The drawing under review shows one solid part. Ordinate dimensions are in mm from its lowest x, y, z. A direction names the side the tool comes from. Coordinates: 2 decimals unless noted, no trailing zeros. Write each loop counter-clockwise with the first axis right and the second up, starting at its lowest first coordinate (ties: lowest second). Pieces come first, ordered by that corner, then holes.
Q1. To check wall thickness, follow probe 1 along Y at (x, z) = (17.5, 8.5); probe 2 along Z at (x, y) = (12.7, 10.7); probe 3 along Y at (x, z) = (12.7, 2.3). State the ranges of each line that lie inside material, in increasing order.
Q2. Add section B-B, the plane x = 15. Give the boundary of the cut face in (y, z) (3 decimals).
Q3. Add section A-A, the plane z = 6.75. Give the boundary of the cut face in (x, y), plus the area to 3 significant figures.
Q4. Clearance check with flat-ended pins moving along their axes: pin 1 Ø4 at (y, z) = (19.5, 3.5) entering from -X; pin 2 Ø8 at (x, z) = (18.5, 11) entering from +Y; pin 3 Ø3 at (y, z) = (18, 6) entering from +X; pin 4 Ø15 at (x, y) = (18, 22) entering from +Z (3 decimals). State where each tip first meets the part, or that it passes through.
Q5. Machinability: for the marked faces 1, 2 and 3, which of the approach directions +Z, -Z, +X, -X, +Y, -Y give a long, thin tool a straight path to every point of the face, cutting with its end or side? Answer none if there is none.
Q6. Add section D-D, the plane z = 14.25. Give the boundary of the cut face in (x, y).
Q7. The part is to be moulded in two halves that separate along X. For the marked faces 4, 5, 6 and 7, say which applies: +X half, -X half, draft (parallel to the pull), parting line (faces both ways), or undercut.
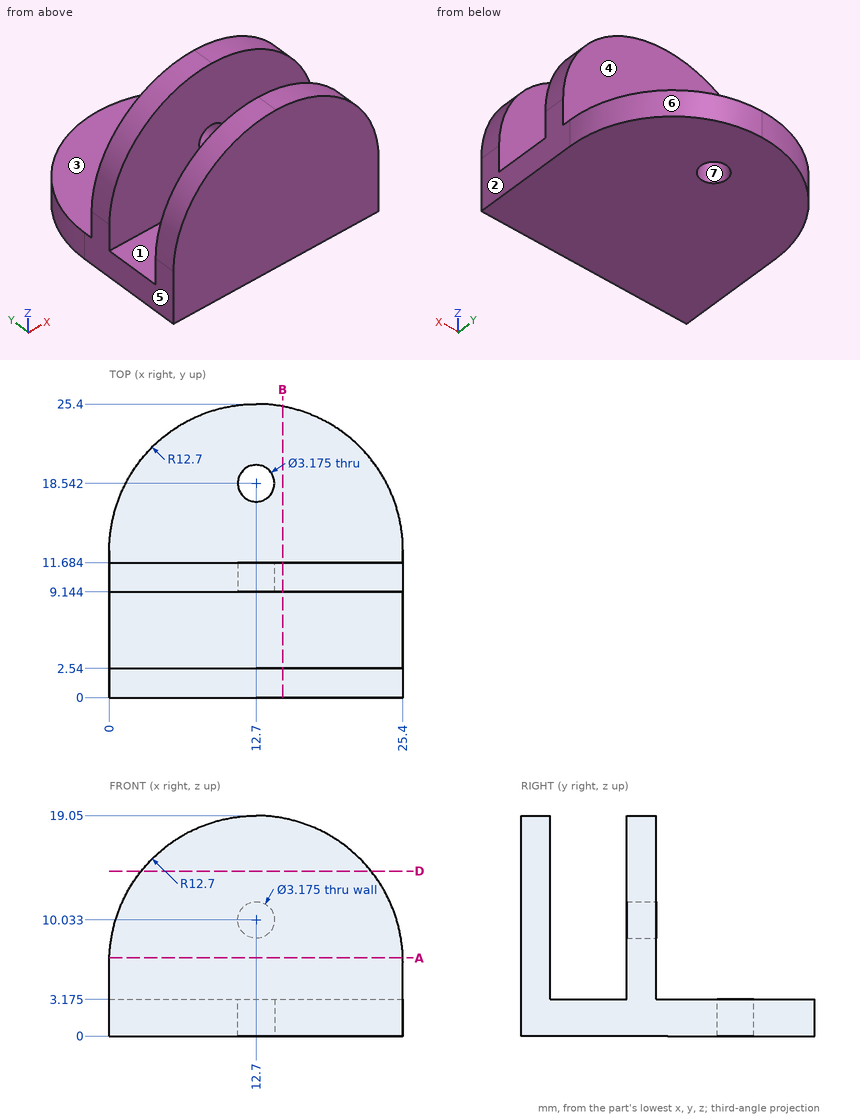
Here are the results:
1. probe 1: y = 0 to 2.54, 9.14 to 11.68
1. probe 2: z = 0 to 8.45, 11.62 to 19.05
1. probe 3: y = 0 to 16.95, 20.13 to 25.4
2. outline: (0, 0) - (25.19, 0) - (25.19, 3.175) - (11.684, 3.175) - (11.684, 18.84) - (9.144, 18.84) - (9.144, 3.175) - (2.54, 3.175) - (2.54, 18.84) - (0, 18.84) - close
3. outline: (0.01, 0) - (25.39, 0) - (25.39, 2.54) - (0.01, 2.54) - close; (0.01, 9.14) - (25.39, 9.14) - (25.39, 11.68) - (0.01, 11.68) - close
3. area: 129 mm2
4. pin 1: stops at x = 0.95
4. pin 2: stops at y = 11.68
4. pin 3: passes through
4. pin 4: stops at z = 3.175
5. face 1: +Z, +X, -X
5. face 2: +Z, -Z, +X, +Y, -Y
5. face 3: +Z, +X, -X, +Y
6. outline: (2.76, 0) - (22.64, 0) - (22.64, 2.54) - (2.76, 2.54) - close; (2.76, 9.14) - (22.64, 9.14) - (22.64, 11.68) - (2.76, 11.68) - close
7. face 4: draft
7. face 5: -X half
7. face 6: +X half
7. face 7: undercut
